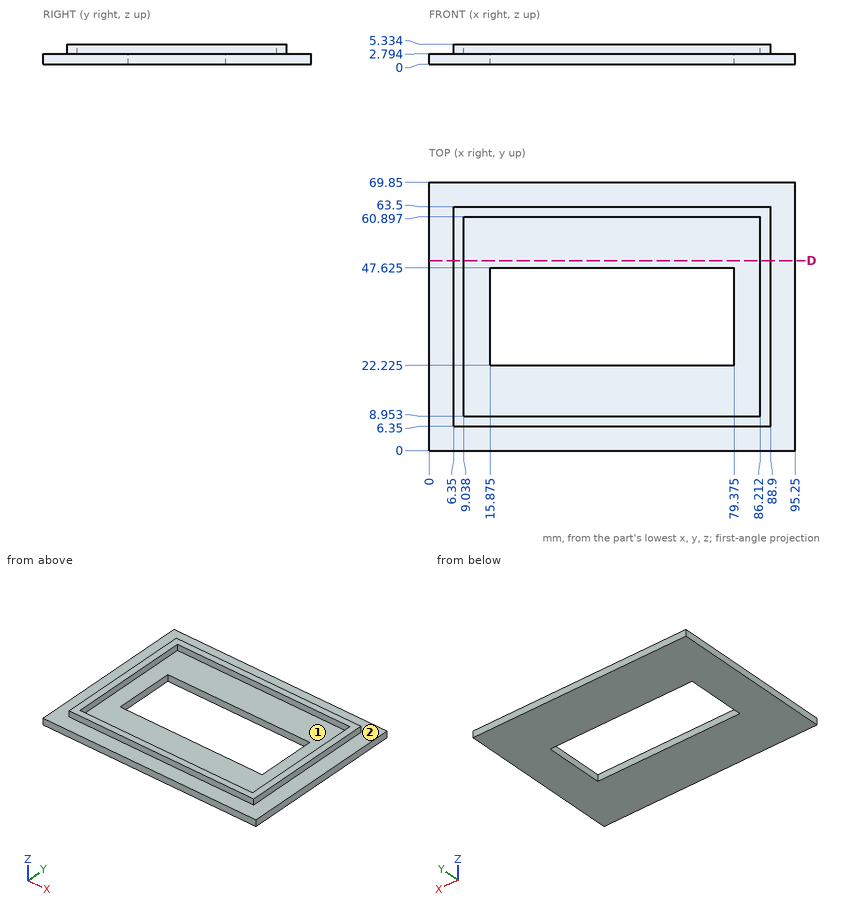
Geometry: see drawing. Coordinates: mm, zero at the bounding-box minimum. Coordinates: 2 decimals unless noted, no trailing zeros. Order: outer loops, then holes, each group sorted by start corner. A loop starts at its lowest first (then second) coordinate and runs counter-clockwise, first axis right, second up. Notation, with made-up numbers: (0, 58.25) - (4, 58.25) arc R12 ccw to (4, 77.25) - close; hole circle Ø8 at (30.5, 80). An arc over 180 degrees is marked (long way). Write each question's results on one line, items separated by ' | '.
(1) Section query D-D, the plane y = 49.5. Return the cut outline in (x, z).
Values found:
outline: (0, 0) - (95.25, 0) - (95.25, 2.79) - (88.9, 2.79) - (88.9, 5.33) - (86.21, 5.33) - (86.21, 2.79) - (9.04, 2.79) - (9.04, 5.33) - (6.35, 5.33) - (6.35, 2.79) - (0, 2.79) - close
(2) First-contact query: pin 1 Ø1.3 at (x, z) = (64.5, 4) entering from +Y; pin 2 Ø1.3 at (x, z) = (28.5, 4) entering from -Y; pin 3 Ø5 at (x, y) = (67.5, 18) entering from +Z. Flat tips, straight axial feed; report the tip coordinate or a pass-through.
Values found:
pin 1: stops at y = 63.5 | pin 2: stops at y = 6.35 | pin 3: stops at z = 2.79
(3) Mould query, pull axis Y, two halves, no side actions, for the marked faces 1 and 2. Classes: +Y half, -Y half, draft (parallel to the pull), parting line (faces both ways), or undercut.
Values found:
face 1: undercut | face 2: draft
(4) Line query: line 1 (Y direction, x = 39.5, z = 3); line 2 (X direction, y = 47, z = 5); line 3 (X direction, y = 62, z = 4.25). Output: solid intervals per line, ascending. Write a range as [from, to].
Values found:
line 1: y = [6.35, 8.95], [60.9, 63.5] | line 2: x = [6.35, 9.04], [86.21, 88.9] | line 3: x = [6.35, 88.9]
